Answer from the drawing. Dimensions are ordinates in mm from the lowest x, y and z of the part. A direction names the side the tool comes from. Coordinates: 2 decimals unless noted, no trailing zeros. Order: outer loops, then holes, each group sorted by start corner. A loop starts at its lowest first (then second) coordinate and runs counter-clockwise, first axis right, second up. Notation, with made-up numbers: (-29, 17) - (26, 17) arc R21 ccw to (26, 47) - close; hole circle Ø2 at (34.25, 59.25). An arc over 180 degrees is marked (long way). Answer as a JSON object with one key per item and string values. Group by question number.
1) The mould has two halves that part along X. Classify the marked faces 3, 4 and 5: released by +X, released by -X, zero draft, split by the parting line, or undercut.
2) Section D-D (y = 58) is taken. Give the vertices of the cut face in (x, z).
3) Section A-A (x = 25) is taken. Give the vertices of the cut face in (y, z) (1 decimal), plus the area to 3 significant figures.
4) Section B-B (y = 48.5) is taken. Give the vertices of the cut face in (x, z), plus the area to 3 significant figures.
5) Find the intervals of material crossed by line 1 along X through (y, z) = (56.5, 26) (1 decimal); line 2 along X through (y, z) = (64, 37.5); line 3 along Y through (x, z) = (43.5, 27) (1 decimal), in increasing order.
6) A tool of negligible diameter and unlimited length cuts with its end or side. For the marked faces 1 and 2, from which of +Z, -Z, +X, -X, +Y, -Y can it reach the whole face along a straight path? Write none if from no direction.
7) Section C-C (z = 17) is taken. Count the separate pieces of the cut face and the enclosed holes in it, plus the area to 3 significant figures.
8) Each of these flat-tipped pins is pushed along its axis until it touches: P1, Ø1.5, axis at x = 10, y = 44.5, coming from the +Z side; P2, Ø3, axis at x = 43.5, z = 31, coming from the -Y side; P3, Ø2, axis at x = 32, y = 73.5, coming from the +Z side. Where does it stop, or does it pass through?
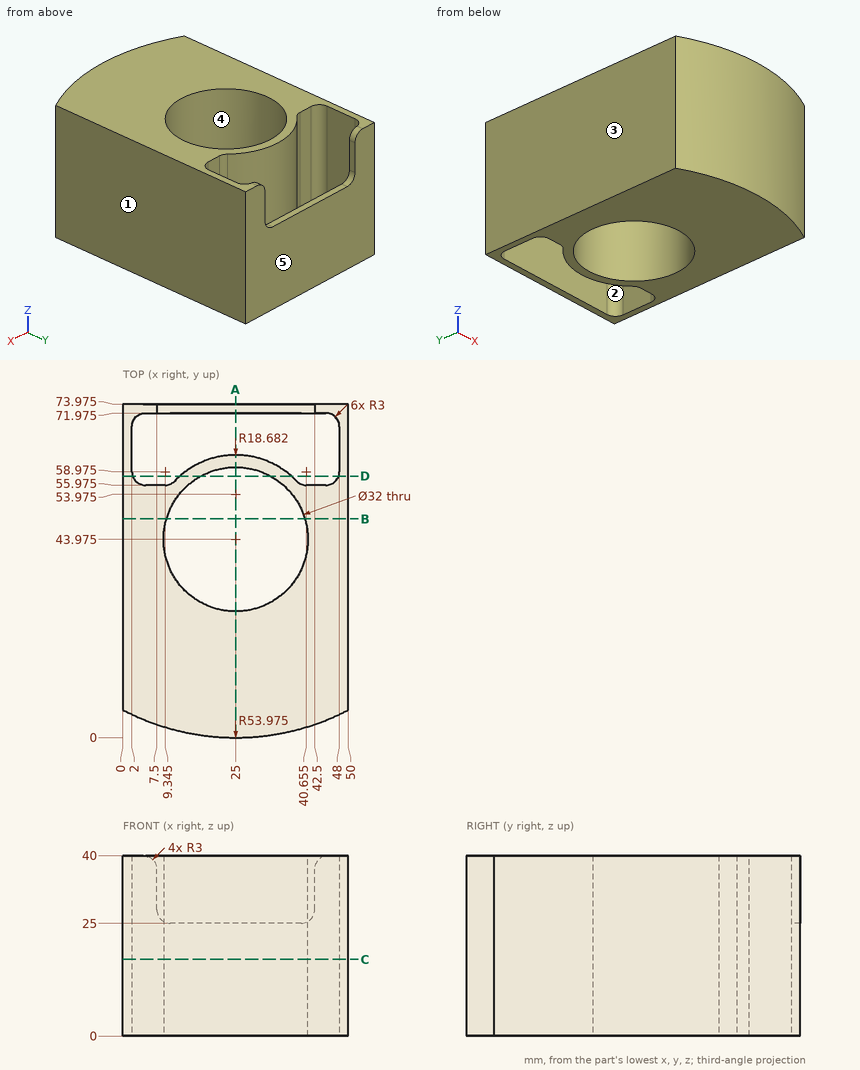
Report:
{
 "1": {"face 3": "released by -X", "face 4": "undercut", "face 5": "zero draft"},
 "2": {"outline": "(0, 0) - (2.16, 0) - (2.16, 40) - (0, 40) - close; (12.66, 0) - (17.3, 0) - (17.3, 40) - (12.66, 40) - close; (32.7, 0) - (37.34, 0) - (37.34, 40) - (32.7, 40) - close; (47.84, 0) - (50, 0) - (50, 40) - (47.84, 40) - close"},
 "3": {"outline": "(0, 0) - (28, 0) - (28, 40) - (0, 40) - close; (60, 0) - (62.7, 0) - (62.7, 40) - (60, 40) - close; (72, 0) - (74, 0) - (74, 25) - (72, 25) - close", "area": "1,280 mm²"},
 "4": {"outline": "(0, 0) - (9.65, 0) - (9.65, 40) - (0, 40) - close; (40.35, 0) - (50, 0) - (50, 40) - (40.35, 40) - close", "area": "772 mm²"},
 "5": {"line 1": "x = 0 to 3.3, 11 to 15, 35 to 39, 46.7 to 50", "line 2": "x = 0 to 2, 48 to 50", "line 3": "y = 3.3 to 56, 72 to 74"},
 "6": {"face 1": "+Z, -Z, +X, +Y, -Y", "face 2": "+Z, -Z"},
 "7": {"separate pieces": "1", "enclosed holes": "2", "area": "2,200 mm²"},
 "8": {"P1": "passes through", "P2": "stops at y = 2.75", "P3": "stops at z = 25"}
}
